For this review, take the finished solid that the model builds, in its own axes (mm). Face numbers are marked on the shaded views. Round coordinates to 2 decimals unless told otherwise and drop trailing zeros. Write each loop counter-clockwise with the first axis right and the second up, starting at its lowest first coordinate (ties: lowest second). Pieces come first, ordered by that corner, then holes. Notation, with made-up numbers: (89, -28) -> (110, -28) arc R25 ccw to (110, 9) -> close; hole circle Ø7 at (-11.5, -35.75). An arc over 180 degrees is marked (long way). Answer as CSV lines item,"result". Start each with the question number.
Item 1: For pin 1 Ø5.5 at (x, z) = (38.5, -0.5) entering from -Y; pin 2 Ø4 at (x, z) = (40, 0) entering from -Y; pin 3 Ø14.5 at (x, z) = (-1, 37) entering from -Y; pin 4 Ø10 at (x, y) = (11, -20) entering from -Z, all flat-tipped, find the tip position at first contact; note any pin that passes through.
Item 2: Take a section at A-A on x = 0. Give the boundary of the cut face in (y, z).
Item 3: Mouldability with a two-part tool opening along X and no side actions: class the marked faces 1, 2 and 3 as +X half, -X half, draft (parallel to the pull), parting line (faces both ways), or undercut.
Item 4: Take a section at B-B on z = 0. Give the boundary of the cut face in (x, y), then the cut area to 3 significant figures.
Item 5: Wall thickness on probe 1 along X at (y, z) = (2, 0); probe 2 along X at (y, z) = (-2, 13); probe 3 along X at (y, z) = (-8.5, -8): over which ranges is each line inside the solid? List them lowest first. Write a range as from..to.
Item 6: Take a section at D-D on y = -8.5. Give the boundary of the cut face in (x, z), then the cut area to 3 significant figures.
Item 7: Take a section at C-C on z = 40. Give the boundary of the cut face in (x, y).
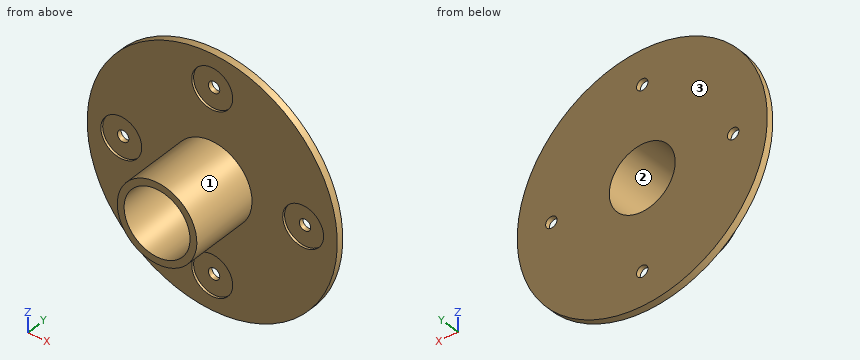
```python
from build123d import *

# Parameters (mm, degrees)
SKETCH1_R           = 55
BOSS_EXTRUDE1_DEPTH = 3
SKETCH2_R           = 17.5
BOSS_EXTRUDE2_DEPTH = 30
SKETCH3_R           = 14.5
CUT_EXTRUDE1_DEPTH  = 85.492603227
SKETCH4_R           = 2.5
CUT_EXTRUDE2_DEPTH  = 85.492603227
SKETCH5_R           = 9
CUT_EXTRUDE3_DEPTH  = 1


with BuildPart() as part:
    # Sketch1 → Boss-Extrude1 (new body)
    with BuildSketch(Plane(origin=(0, 0, 0), x_dir=(1, 0, 0), z_dir=(0, 1, 0))):
        with Locations(Location((0, 0, 0), (0, 0, 270))):
            Circle(SKETCH1_R)
    extrude(amount=BOSS_EXTRUDE1_DEPTH)

    # Sketch2 → Boss-Extrude2 (add)
    with BuildSketch(Plane.XZ):
        with Locations(Location((0, 0, 0), (0, 0, 270))):
            Circle(SKETCH2_R)
    extrude(amount=BOSS_EXTRUDE2_DEPTH)

    # Sketch3 → Cut-Extrude1 (cut, through all)
    with BuildSketch(Plane.XZ.offset(30)):
        with Locations(Location((0, 0, 0), (0, 0, 270))):
            Circle(SKETCH3_R)
    extrude(amount=-CUT_EXTRUDE1_DEPTH, mode=Mode.SUBTRACT)

    # Sketch4 → Cut-Extrude2 (cut, through all)
    with BuildSketch(Plane(origin=(0, 3, 0), x_dir=(1, 0, 0), z_dir=(0, 1, 0))):
        with Locations(Location((0, 40, 0), (0, 0, 270))):
            Circle(SKETCH4_R)
        with Locations(Location((40, 0, 0), (0, 0, 270))):
            Circle(SKETCH4_R)
        with Locations(Location((0, -40, 0), (0, 0, 270))):
            Circle(SKETCH4_R)
        with Locations(Location((-40, 0, 0), (0, 0, 270))):
            Circle(SKETCH4_R)
    extrude(amount=-CUT_EXTRUDE2_DEPTH, mode=Mode.SUBTRACT)

    # Sketch5 → Cut-Extrude3 (cut)
    with BuildSketch(Plane.XZ):
        with Locations(Location((0, 40, 0), (0, 0, 270))):
            Circle(SKETCH5_R)
        with Locations(Location((40, 0, 0), (0, 0, 270))):
            Circle(SKETCH5_R)
        with Locations(Location((0, -40, 0), (0, 0, 270))):
            Circle(SKETCH5_R)
        with Locations(Location((-40, 0, 0), (0, 0, 270))):
            Circle(SKETCH5_R)
    extrude(amount=-CUT_EXTRUDE3_DEPTH, mode=Mode.SUBTRACT)


solid = part.part
```
Output values:
1,pin 1,"stops at y = 1"
1,pin 2,"passes through"
1,pin 3,"stops at y = 0"
1,pin 4,"stops at z = -16.44"
2,outline,"(-30, -17.5) -> (0, -17.5) -> (0, -31) -> (1, -31) -> (1, -37.5) -> (3, -37.5) -> (3, -14.5) -> (-30, -14.5) -> close; (-30, 14.5) -> (3, 14.5) -> (3, 37.5) -> (1, 37.5) -> (1, 31) -> (0, 31) -> (0, 17.5) -> (-30, 17.5) -> close; (0, -55) -> (3, -55) -> (3, -42.5) -> (1, -42.5) -> (1, -49) -> (0, -49) -> close; (0, 49) -> (1, 49) -> (1, 42.5) -> (3, 42.5) -> (3, 55) -> (0, 55) -> close"
3,face 1,"parting line"
3,face 2,"undercut"
3,face 3,"draft"
4,outline,"(-55, 0) -> (-49, 0) -> (-49, 1) -> (-42.5, 1) -> (-42.5, 3) -> (-55, 3) -> close; (-37.5, 1) -> (-31, 1) -> (-31, 0) -> (-17.5, 0) -> (-17.5, -30) -> (-14.5, -30) -> (-14.5, 3) -> (-37.5, 3) -> close; (14.5, -30) -> (17.5, -30) -> (17.5, 0) -> (31, 0) -> (31, 1) -> (37.5, 1) -> (37.5, 3) -> (14.5, 3) -> close; (42.5, 1) -> (49, 1) -> (49, 0) -> (55, 0) -> (55, 3) -> (42.5, 3) -> close"
4,area,"367 mm^2"
5,probe 1,"x = -55..-42.5, -37.5..-14.5, 14.5..37.5, 42.5..55"
5,probe 2,"x = -11.72..-6.42, 6.42..11.72"
5,probe 3,"x = -15.56..-12.09, 12.09..15.56"
6,outline,"circle Ø35 at (0, 0); hole circle Ø29 at (0, 0)"
6,area,"302 mm^2"
7,outline,"(-37.75, 0) -> (-9, 0) -> (-9, 1) -> (-2.5, 1) -> (-2.5, 3) -> (-37.75, 3) -> close; (2.5, 1) -> (9, 1) -> (9, 0) -> (37.75, 0) -> (37.75, 3) -> (2.5, 3) -> close"
